Autodesk Inventor part; units mm, degrees
ref_plane "YZ Plane" through (0, 0, 0) normal (1, 0, 0) x (0, 1, 0)
ref_plane "XZ Plane" through (0, 0, 0) normal (0, 1, 0) x (-1, 0, 0)
ref_plane "XY Plane" through (0, 0, 0) normal (0, 0, 1) x (1, 0, 0)
sketch "Sketch1" plane through (0, 0, 0) normal (0, 0, 1) x (1, 0, 0)
  line L0 (-13.5, 6) -> (13.5, 6)
  line L1 (13.5, 6) -> (13.5, -6)
  line L2 (13.5, -6) -> (-13.5, -6)
  line L3 (-13.5, -6) -> (-13.5, 6)
  line L4 (-8.625, -6) -> (-8.625, 2)
  line L5 (-8.625, 2) -> (8.625, 2)
  line L6 (8.625, 2) -> (8.625, -6)
  line L7 (0, 19.1515) -> (0, -21.0963) construction
  line L8 (-12.5, -6) -> (-12.5, 5)
  line L9 (-12.5, 5) -> (12.5, 5)
  line L10 (12.5, 5) -> (12.5, -6)
  circle A0 centre (10.625, -3) radius 1.25
  circle A1 centre (-10.625, -3) radius 1.25
  line L11 (10.625, -5.3094) -> (8.625, -4.1547)
  line L12 (8.625, -4.1547) -> (8.625, -1.8453)
  line L13 (8.625, -1.8453) -> (10.625, -0.6906)
  line L14 (10.625, -0.6906) -> (12.625, -1.8453)
  line L15 (12.625, -1.8453) -> (12.625, -4.1547)
  line L16 (12.625, -4.1547) -> (10.625, -5.3094)
  line L17 (-10.625, -5.3094) -> (-12.625, -4.1547)
  line L18 (-12.625, -4.1547) -> (-12.625, -1.8453)
  line L19 (-12.625, -1.8453) -> (-10.625, -0.6906)
  line L20 (-10.625, -0.6906) -> (-8.625, -1.8453)
  line L21 (-8.625, -1.8453) -> (-8.625, -4.1547)
  line L22 (-8.625, -4.1547) -> (-10.625, -5.3094)
  line L23 (13.5, 6) -> (13.5, 17)
  line L24 (13.5, 17) -> (-13.5, 17)
  line L25 (-13.5, 17) -> (-13.5, 6)
  point P0 (0, 0)
  point P1 (-13.5, 0)
  point P2 (0, 6)
  point P3 (0, 16)
  dimension "d2" = 17.25
  dimension "d3" = 1
  dimension "d4" = 1
  dimension "d5" = 3
  dimension "d10" = 2.5
  dimension "d11" = 21.25
  dimension "d12" = 8
  dimension "d13" = 2
  dimension "d16" = 11
  dimension "d17" = 25
  dimension "d19" = 15
extrude "body" add sketch "Sketch1" along normal blind 2 contours L0 L1 L2 L10 L16 L15 L14 L9 L8 L19 L18 L17 L3 | L8 L17 L22 L4 L2 | L2 L6 L11 L16 L10 | L17 L18 L19 L8 | L8 L19 L20 L4 L22 L17 | L16 L11 L6 L13 L14 L10 | L10 L14 L15 L16 | L8 L9 L10 L14 L13 L6 L5 L4 L20 L19
extrude "borders" add sketch "Sketch1" along normal blind 4 contours L0 L1 L2 L10 L16 L15 L14 L9 L8 L19 L18 L17 L3 | L17 L18 L19 L8 | L10 L14 L15 L16
extrude "nut_recesses" [suppressed]
extrude "jut out for imu" add sketch "Sketch1" along normal blind 2.5 contours L25 L24 L23 L0
sketch "Sketch2" plane through (0, 0, 2.5) normal (0, 0, 1) x (1, 0, 0)
  line L0 (-10.5, 20) -> (10.5, 20)
  line L1 (10.5, 20) -> (10.5, 6.5)
  line L2 (10.5, 6.5) -> (-10.5, 6.5)
  line L3 (-10.5, 6.5) -> (-10.5, 20)
  circle A0 centre (-8, 9) radius 1.25
  line L4 (13.5, 6) -> (-13.5, 6)
  line L5 (10.23, 6.5) -> (10.23, 20)
  line L6 (8.23, 20) -> (8.23, 6.5)
  line L7 (8.23, 13.25) -> (10.23, 13.25) construction
  point P0 (0, 0)
  point P1 (0, 20)
  point P2 (9.23, 13.25)
  dimension "d32" = 21
  dimension "d33" = 13.5
  dimension "d34" = 2.5
  dimension "d35" = 2.5
  dimension "d36" = 2.5
  dimension "d44" = 0.5
  dimension "d45" = 2
  dimension "d46" = 1.27
extrude "recess for imu" cut sketch "Sketch2" along normal blind 10 and the other way blind 1 contours L0 L6 L2 L3 | L0 L5 L2 L6 | L0 L1 L2 L5 | A0
extrude "hole for imu" cut sketch "Sketch2" against normal blind 10 contours A0
fillet "Fillet2" radius 1 3 edges at (-13.5, 5.5, 0) (0, 17, 0) (13.5, 5.5, 0)
extrude "Extrusion9" cut sketch "Sketch2" against normal blind 2 contours L0 L5 L2 L6
equation "\"d4\" = d3"
properties part number "imu_mount"
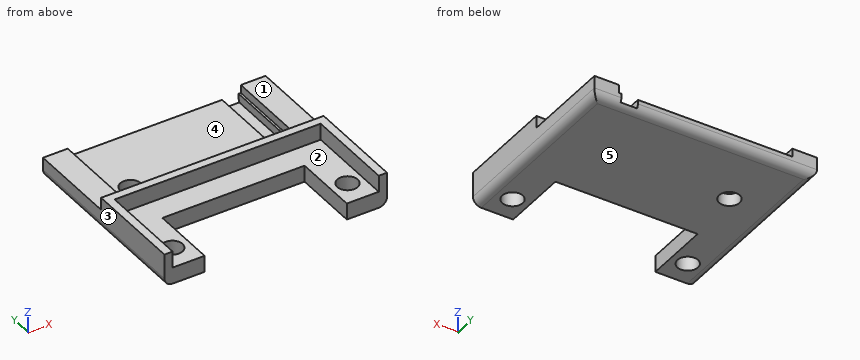
Geometry: final body of the model. Coordinates: model frame, mm. Face numbers are marked on the shaded views. A direction names the side the tool comes from. Coordinates: 2 decimals unless noted, no trailing zeros. Order: outer loops, then holes, each group sorted by start corner. A loop starts at its lowest first (then second) coordinate and runs counter-clockwise, first axis right, second up.
1) Section A-A (x = -8). Return loops of the section in (y, z).
Result sheet:
outline: (2, 0) - (7.75, 0) - (7.75, 1.5) - (6.5, 1.5) - (6.5, 2.5) - (6, 2.5) - (6, 4) - (5, 4) - (5, 2) - (2, 2) - close; (10.25, 0) - (16, 0) arc R1 ccw to (17, 1) - (17, 1.5) - (10.25, 1.5) - close
2) Draft query along X for the marked faces 1, 2 and 3. Return one class per face: released by +X, released by -X, zero draft, split by the parting line, or undercut.
Result sheet:
face 1: zero draft
face 2: undercut
face 3: released by -X
3) Section B-B (y = 9). Return loops of the section in (x, z).
Result sheet:
outline: (-13.5, 1) arc R1 ccw to (-12.5, 0) - (-9.25, 0) - (-9.25, 1.5) - (-10.5, 1.5) - (-10.5, 2.5) - (-13.5, 2.5) - close; (-6.75, 0) - (12.5, 0) arc R1 ccw to (13.5, 1) - (13.5, 2.5) - (10.5, 2.5) - (10.5, 1.5) - (10.23, 1.5) - (10.23, 0.5) - (8.23, 0.5) - (8.23, 1.5) - (-6.75, 1.5) - close
4) Ray query, probe 1 along X at (y, z) = (-3.5, 3.7); probe 2 along X at (y, z) = (13.75, 1.25); probe 3 along Z at (x, y) = (6.25, 3.5). Return the intervals inside material, ascending.
Result sheet:
probe 1: x = -13.5 to -12.5, 12.5 to 13.5
probe 2: x = -13.5 to 8.23, 10.23 to 13.5
probe 3: z = 0 to 2
5) Section C-C (y = -3). Return loops of the section in (x, z) (3 decimals).
Result sheet:
outline: (-13.5, 1) arc R1 ccw to (-12.5, 0) - (-11.875, 0) - (-11.875, 2) - (-12.5, 2) - (-12.5, 4) - (-13.5, 4) - close; (-9.375, 0) - (-8.625, 0) - (-8.625, 2) - (-9.375, 2) - close; (8.625, 0) - (9.375, 0) - (9.375, 2) - (8.625, 2) - close; (11.875, 0) - (12.5, 0) arc R1 ccw to (13.5, 1) - (13.5, 4) - (12.5, 4) - (12.5, 2) - (11.875, 2) - close
6) Section D-D (x = 7.75). Return loops of the section in (y, z).
Result sheet:
outline: (2, 0) - (16, 0) arc R1 ccw to (17, 1) - (17, 1.5) - (6.5, 1.5) - (6.5, 2.5) - (6, 2.5) - (6, 4) - (5, 4) - (5, 2) - (2, 2) - close
7) Set-up query: the marked faces 4 and 5. Return all of +Z, -Z, +X, -X, +Y, -Y with unobstructed straight access to the full face (end or side cutting, diameter ignored); none if empty.
Result sheet:
face 4: +Z, +Y
face 5: -Z, +X, -X, +Y, -Y
8) First-contact query: P1, Ø0.8, axis at x = 1, z = 3.5, coming from the +Y side; P2, Ø12, axis at x = 8, y = 12.5, coming from the +Z side; P3, Ø12, axis at x = -5, y = -3, coming from the +Z side. Flat tips, straight axial feed; report the tip coordinate or a pass-through.
Result sheet:
P1: stops at y = 6
P2: stops at z = 2.5
P3: stops at z = 2
